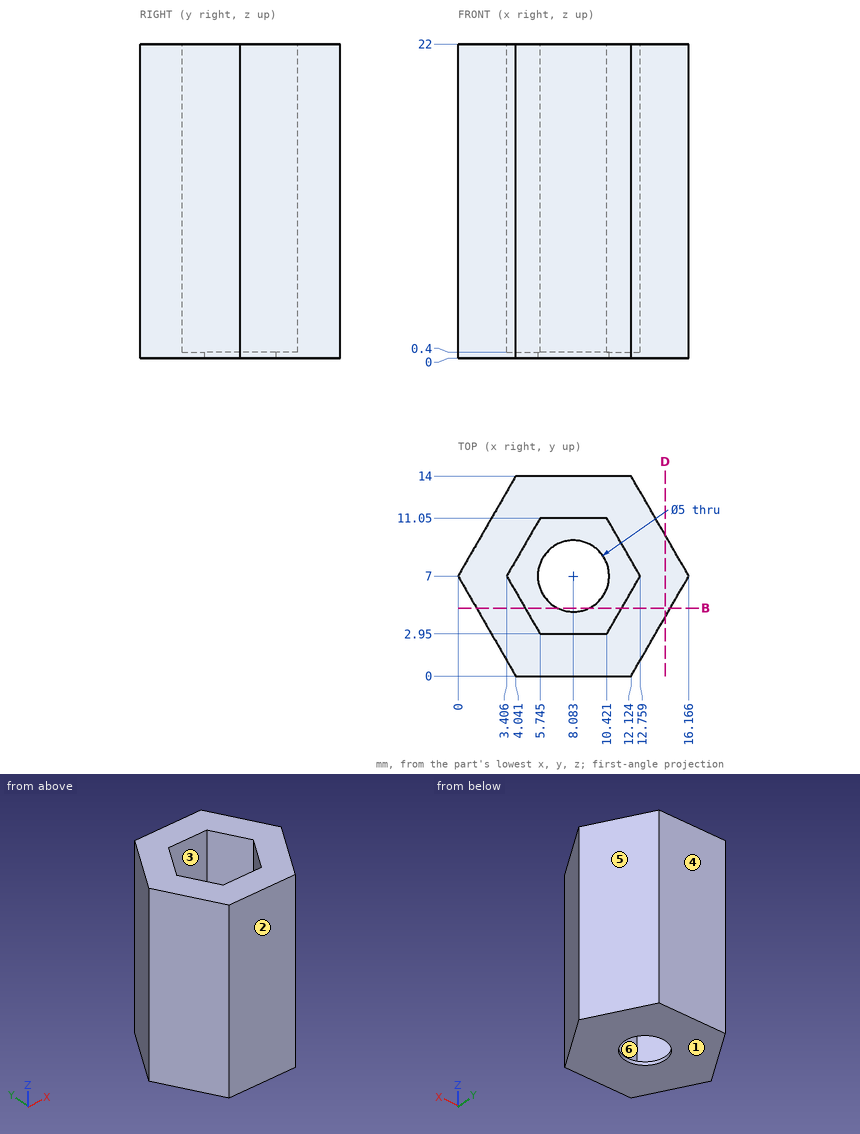
Here's the drawing with two shaded views (mm, measured from the low corner). I have some questions. A direction names the side the tool comes from. Coordinates: 2 decimals unless noted, no trailing zeros. Write each loop counter-clockwise with the first axis right and the second up, starting at its lowest first coordinate (ties: lowest second). Pieces come first, ordered by that corner, then holes. Notation, with made-up numbers: (31.5, 50.25) -> (44.5, 50.25) arc R10 ccw to (44.5, 58.25) -> close; hole circle Ø6 at (17, 48). An arc over 180 degrees is marked (long way). One line per question, with ' | ' between items. Start each with the question number.
1. If we section it at D-D (x = 14.5): Please give me the cut outline in (y, z) (1 decimal).
2. Please list where these lines run through material, in increasing order: line 1 along Y through (x, z) = (8.75, 19.25); line 2 along Z through (x, y) = (10.5, 4); line 3 along X through (y, z) = (9.25, 10.5) (1 decimal).
3. Thinking about a two-plate mould opening in Y: for the marked faces 1, 2, 3 and 4, which applies, pulls with the +Y half, pulls with the -Y half, needs draft (parallel to the pull), parting line crosses it, or undercut?
4. Will these pins go through, and if not, where does the flat tip stop? P1, Ø6, axis at x = 8.08, y = 7, coming from the +Z side; P2, Ø4, axis at y = 4, z = 17, coming from the -X side; P3, Ø1, axis at y = 2, z = 9, coming from the +X side.
5. If we section it at B-B (y = 4.75): Please give me the cut outline in (x, z) (1 decimal).
6. For the marked faces 5 and 6, which set-ups out of +Z, -Z, +X, -X, +Y, -Y let a thin tool reach every point of the face, with its end or its side?
Return value:
1) outline: (4.1, 0) -> (9.9, 0) -> (9.9, 22) -> (4.1, 22) -> close
2) line 1: y = 0 to 2.95, 11.05 to 14 | line 2: z = 0 to 0.4 | line 3: x = 1.3 to 4.7, 11.5 to 14.9
3) face 1: needs draft | face 2: pulls with the -Y half | face 3: undercut | face 4: pulls with the +Y half
4) P1: stops at z = 0.4 | P2: stops at x = 0.58 | P3: stops at x = 13.57
5) outline: (1.3, 0) -> (7, 0) -> (7, 0.4) -> (4.7, 0.4) -> (4.7, 22) -> (1.3, 22) -> close; (9.2, 0) -> (14.9, 0) -> (14.9, 22) -> (11.5, 22) -> (11.5, 0.4) -> (9.2, 0.4) -> close
6) face 5: +Z, -Z, +X, +Y | face 6: +Z
